Geometry: see drawing. Coordinates: mm, zero at the bounding-box minimum. A direction names the side the tool comes from. Give positions to 0.01 mm unless a question says otherwise; leave off trailing zeros. Write each loop counter-clockwise with the first axis right and the second up, starting at its lowest first coordinate (ties: lowest second). Pieces come first, ordered by that corner, then holes. Notation, with made-up numbers: M 1.25,24.25 L 8.25,24.25 A10 cw 8.25,37.25 Z; hole C 74,-28.5 d7. An arc over 180 degrees is marked long. Use a Markdown table: item, result. Add a question column.
(1) Pin query (flat end, axial travel): pin 1 Ø4.5 at (x, y) = (6, 4) entering from -Z; pin 2 Ø2.5 at (x, y) = (8, 12) entering from +Z; pin 3 Ø1.5 at (x, y) = (3, 6.5) entering from +Z. Return the tip coordinate at first contact, or that it passes through.
(2) Cut plane C-C (z = 0.25). Output: boundary loops of the cut face in (x, y).
(3) Cut plane A-A (x = 6). Output: boundary loops of the cut face in (y, z).
(4) Cut plane D-D (z = 3.5). Output: boundary loops of the cut face in (x, y).
(5) Draft query along X for the marked faces 1, 2 and 3. Return one class per face: released by +X, released by -X, zero draft, split by the parting line, or undercut.
(6) Cut plane B-B (y = 4). Output: boundary loops of the cut face in (x, z).
(7) Reachability of the marked faces 4 and 5 from +Z, -Z, +X, -X, +Y, -Y: full face, straight path, thin tool, end or side. Return the list, or none.
(8) Material intervals for L1, parallel to Y at x = 6, z = 1.05; L2, parallel to X at y = 12.25, z = 3.6; L3, parallel to X at y = 4.75, z = 3.3, sorted ascending.
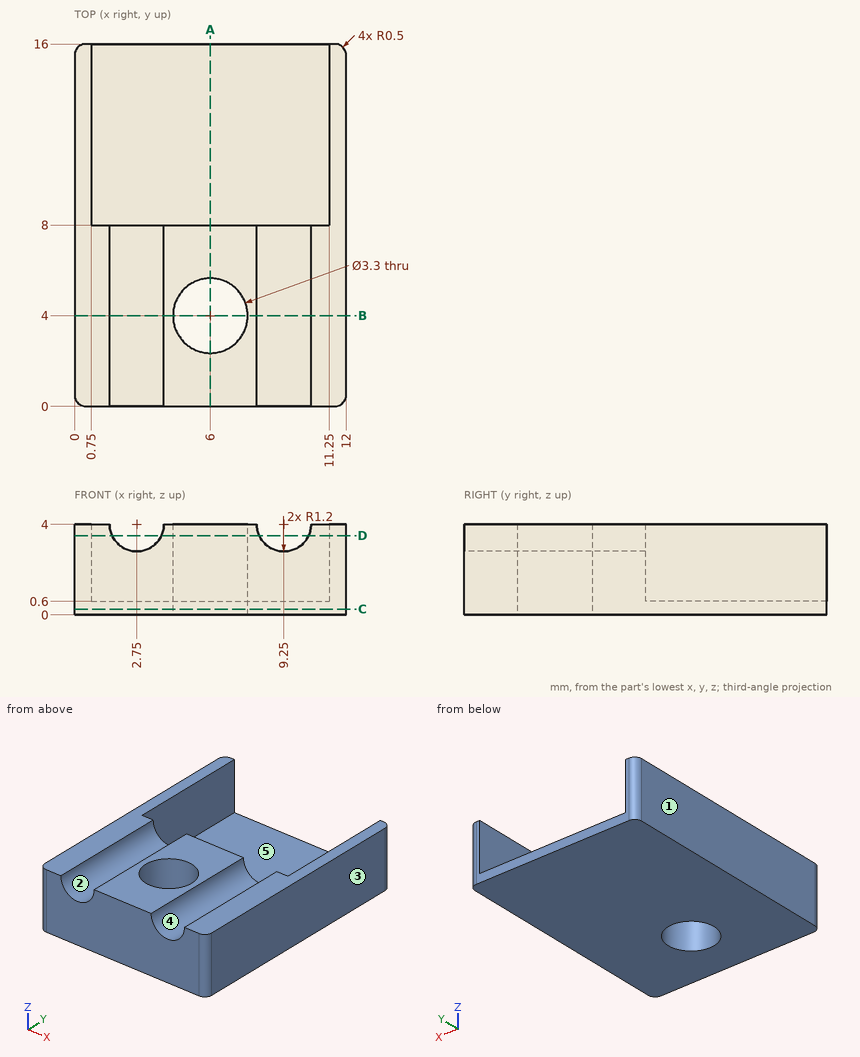
Answer list:
| question | item | result |
|---|---|---|
| 1 | pin 1 | z = 0 |
| 1 | pin 2 | z = 0.6 |
| 1 | pin 3 | z = 3.34 |
| 2 | outline | M 0,0.5 A0.5 ccw 0.5,0 L 11.5,0 A0.5 ccw 12,0.5 L 12,15.5 A0.5 ccw 11.5,16 L 0.5,16 A0.5 ccw 0,15.5 Z; hole C 6,4 d3.3 |
| 3 | outline | M 0,0 L 2.35,0 L 2.35,4 L 0,4 Z; M 5.65,0 L 16,0 L 16,0.6 L 8,0.6 L 8,4 L 5.65,4 Z |
| 4 | outline | M 0,0.5 A0.5 ccw 0.5,0 L 1.66,0 L 1.66,8 L 0.75,8 L 0.75,16 L 0.5,16 A0.5 ccw 0,15.5 Z; M 3.84,0 L 8.16,0 L 8.16,8 L 3.84,8 Z; M 10.34,0 L 11.5,0 A0.5 ccw 12,0.5 L 12,15.5 A0.5 ccw 11.5,16 L 11.25,16 L 11.25,8 L 10.34,8 Z; hole C 6,4 d3.3 |
| 5 | face 1 | released by -X |
| 5 | face 2 | undercut |
| 5 | face 3 | released by +X |
| 6 | outline | M 0,0 L 4.35,0 L 4.35,4 L 3.95,4 A1.2 cw 1.55,4 L 0,4 Z; M 7.65,0 L 12,0 L 12,4 L 10.45,4 A1.2 cw 8.05,4 L 7.65,4 Z |
| 7 | face 4 | +Z, +Y, -Y |
| 7 | face 5 | +Z, +Y |
| 8 | L1 | 0 to 2.35, 5.65 to 8 |
| 8 | L2 | 0 to 0.75, 11.25 to 12 |
| 8 | L3 | 0 to 1.78, 3.72 to 4.53, 7.47 to 8.28, 10.22 to 12 |
